Check sheet for the drawn part. Datum: minimum x, y, z corner. Units: mm. Give positions to 0.01 mm unless a question says otherwise; leave off trailing zeros. Loops run counter-clockwise (first coordinate to the right, second up) from the corner with the lowest first, then second, coordinate; pieces in that order, holes last.
1. Cross-section at A-A, the plane x = 50. Record the cut outline in (y, z), plus the area to 3 significant figures.
2. Release check for a two-part mould opening along X. For the marked faces 1, 2 and 3 record: +X half, -X half, draft (parallel to the pull), parting line (faces both ways), or undercut.
3. Material ranges on L1, parallel to Y at x = 50, z = 14; L2, parallel to Y at x = 66.5, z = 44; L3, parallel to X at y = 72.5, z = 29, recorded low to high.
4. Go/stop test with flat-tipped pins: pin 1 Ø1 at (y, z) = (18, 43) entering from +X; pin 2 Ø2 at (x, z) = (17, 10) entering from +Y; pin 3 Ø1.5 at (x, y) = (80.5, 15) entering from -Z. Record where each tip stops, or that it passes through.
5. Cross-section at C-C, the plane z = 23. Record the cut outline in (x, y).
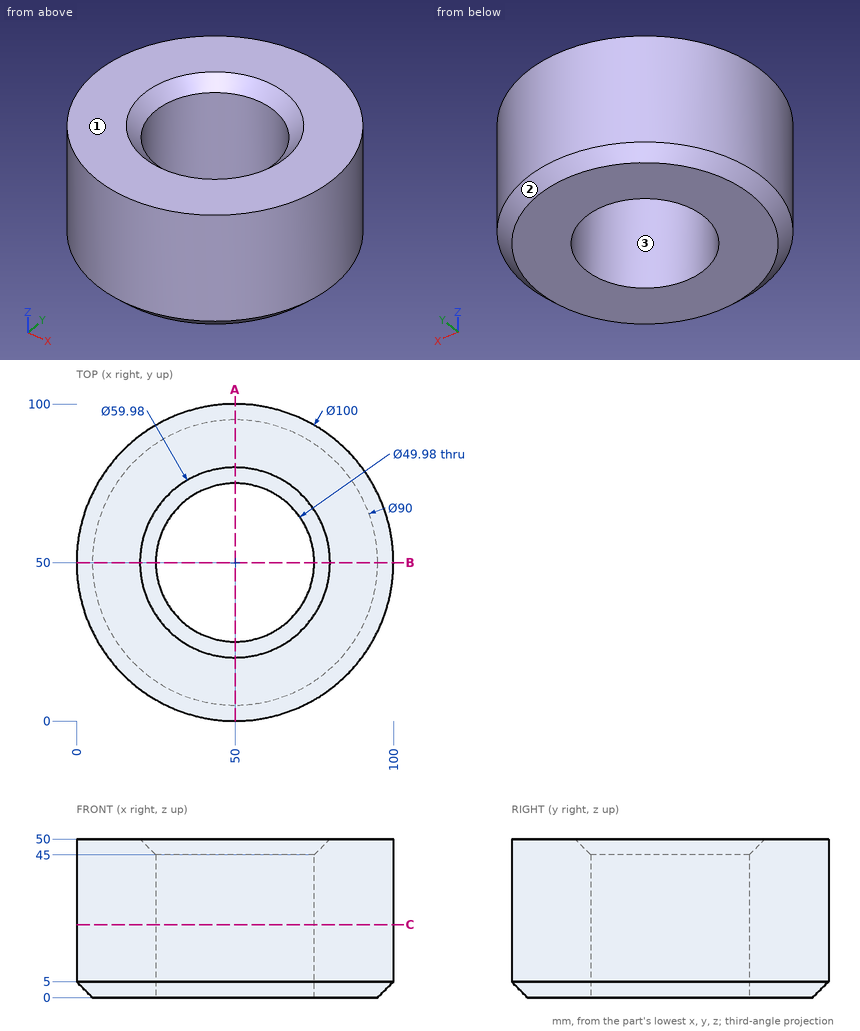
Result:
1. outline: (0, 5) - (5, 0) - (25.01, 0) - (25.01, 45) - (20.01, 50) - (0, 50) - close; (74.99, 0) - (95, 0) - (100, 5) - (100, 50) - (79.99, 50) - (74.99, 45) - close
1. area: 2,450 mm2
2. face 1: draft
2. face 2: parting line
2. face 3: undercut
3. L1: y = 0 to 25.01, 74.99 to 100
3. L2: y = 2.8 to 31.23, 68.77 to 97.2
3. L3: x = 5.35 to 39.13, 60.87 to 94.65
4. pin 1: stops at x = 88.83
4. pin 2: stops at y = 88.42
4. pin 3: stops at z = 0.67
5. outline: circle Ø100 at (50, 50); hole circle Ø49.98 at (50, 50)
